Autodesk Fusion 360 part; units mm, degrees
sketch "Sketch1" plane through (0, 0, 0) normal (0, 0, 1) x (1, 0, 0)
  line L0 (-44, 15.5) -> (44, 15.5)
  line L1 (44, 15.5) -> (44, -15.5)
  line L2 (-44, -15.5) -> (-44, 15.5)
  line L3 (-44, 15.5) -> (44, -15.5) construction
  line L4 (44, 15.5) -> (-44, -15.5) construction
  circle A0 centre (-25, 0) radius 5
  circle A1 centre (25, 0) radius 5
  line L5 (-44, -15.5) -> (-44, -38.5)
  line L6 (44, -38.5) -> (44, -15.5)
  line L7 (-44, 15.5) -> (44, 15.5)
  line L8 (44, 15.5) -> (44, 28.5)
  line L9 (44, 28.5) -> (-44, 28.5)
  line L10 (-44, 28.5) -> (-44, 15.5)
  line L11 (0, -51.5) -> (-5, -51.5)
  line L12 (0, -51.5) -> (5, -51.5)
  line L13 (-5, -51.5) -> (-5, 15.5)
  line L14 (5, -51.5) -> (5, 15.5)
  line L15 (-37.3007, -49.8711) -> (-10.3733, -67.4184)
  line L16 (37.3007, -49.8711) -> (10.3733, -67.4184)
  arc A2 (-10.3733, -67.4184) -> (10.3733, -67.4184) centre (0, -51.5) ccw
  arc A3 (37.3007, -49.8711) -> (44, -38.5) centre (31, -38.5) ccw
  arc A4 (-44, -38.5) -> (-37.3007, -49.8711) centre (-31, -38.5) ccw
  dimension "d1" = 31
  dimension "d2" = 88
  dimension "d3" = 10
  dimension "d4" = 10
  dimension "d5" = 50
  dimension "d6" = 19
  dimension "d7" = 19
  dimension "d9" = 38
  dimension "d12" = 13
  dimension "d13" = 5
  dimension "d14" = 5
  dimension "d15" = 26
  dimension "d16" = 26
extrude "Extrude1" add sketch "Sketch1" along normal blind 10 contours L0 L1 L2 L5 L6 L7 L11 L12 L13 L14 L15 L16 A2 A3 A4
extrude "Extrude2" add sketch "Sketch1" along normal blind 50 contours L0 L7 L8 L9 L10
extrude "Extrude3" add sketch "Sketch1" along normal blind 50 contours L0 L7 L11 L12 L13 L14
sketch "Sketch2" plane through (0, 0, 50) normal (0, 0, 1) x (-1, 0, 0)
  line L0 (44, -28.5) -> (44, -15.5)
  line L1 (44, -15.5) -> (5, -15.5)
  line L2 (5, -15.5) -> (5, 51.5)
  line L3 (5, 51.5) -> (-5, 51.5)
  line L4 (-5, 51.5) -> (-5, -15.5)
  line L5 (-5, -15.5) -> (-44, -15.5)
  line L6 (-44, -15.5) -> (-44, -28.5)
  line L7 (-44, -28.5) -> (44, -28.5)
  circle A0 centre (19, -18.5) radius 3
  circle A1 centre (-19, -18.5) radius 3
  line L8 (19, -18.5) -> (44, -18.5)
  line L9 (-19, -18.5) -> (-44, -18.5)
  line L10 (44, -18.5) -> (44, -15.5)
  line L11 (19, -15.5) -> (19, -18.5)
  line L12 (-19, -18.5) -> (-19, -15.5)
  line L13 (-19, -18.5) -> (-19, -15.5)
  line L14 (-44, -15.5) -> (-44, -18.5)
  line L15 (44, -18.5) -> (44, -37.5)
  line L16 (44, -37.5) -> (-44, -37.5)
  line L17 (-44, -37.5) -> (-44, -18.5)
  circle A2 centre (0, -37.5) radius 9.5
  circle A3 centre (0, -37.5) radius 19
  arc A4 (24.2693, -37.5) -> (18.4447, -42.06) centre (24.2693, -43.5) ccw
  arc A5 (-18.4447, -42.06) -> (-24.2693, -37.5) centre (-24.2693, -43.5) ccw
  dimension "d23" = 6
  dimension "d24" = 6
  dimension "d25" = 38
  dimension "d26" = 25
  dimension "d31" = 19
  dimension "d32" = 19
  dimension "d33" = 38
  dimension "d35" = 12
  dimension "d36" = 12
extrude "Extrude4" cut sketch "Sketch2" against normal blind 40 contours L0 L1 A0 L8 L10
extrude "Extrude5" cut sketch "Sketch2" against normal blind 40 contours L5 L6 A1 L9 L14
sketch "Sketch3" plane through (0, 0, 50) normal (0, 0, 1) x (-1, 0, 0)
extrude "Extrude6" add sketch "Sketch2" against normal blind 50 contours L7 L15 L16 A3 | L7 L16 A2 A3 | L16 A2 A3 | L16 A3 A4 | L7 L16 L17 A3 | L7 L16 A2 A3 | L16 A3 A5
sketch "Sketch4" plane through (-5, 0, 0) normal (-1, 0, 0) x (0, -1, 0)
  line L0 (-15.5, 10) -> (51.5, 10)
  line L1 (51.5, 10) -> (51.5, 50)
  line L2 (51.5, 50) -> (-15.5, 50)
  line L3 (-15.5, 50) -> (-15.5, 10)
  line L4 (-15.5, 50) -> (51.5, 10)
extrude "Extrude7" cut sketch "Sketch4" against normal blind 85 contours L1 L2 L4
equation "d6 = ( ( 88 - 50 ) / 2 ) * 1 mm"
equation "d9 = ( 19 * 2 ) * 1 mm"
equation "d26 = ( ( 88 - 38 ) / 2 ) * 1 mm"
equation "d33 = ( 19 * 2 ) * 1 mm"
Build history of the part. All positions in model axes, mm. A direction names the side the tool comes from. Coordinates: 2 decimals unless noted, no trailing zeros. Order: outer loops, then holes, each group sorted by start corner. A loop starts at its lowest first (then second) coordinate and runs counter-clockwise, first axis right, second up. Notation, with made-up numbers: (84, 20) - (122, 20) arc R35 ccw to (122, 56) - close; hole circle Ø5 at (13, 43.25). An arc over 180 degrees is marked (long way). Put each result on its own line as item: value.
1. Saw through at C-C (z = 31.5). Write the cut outline in (x, y).
Answer sheet:
outline: (-44, 18.5) - (-22, 18.5) arc R3 ccw to (-19, 15.5) - (-5, 15.5) - (-5, -15.49) - (5, -15.49) - (5, 15.5) - (19, 15.5) arc R3 ccw to (22, 18.5) - (44, 18.5) - (44, 37.5) - (24.27, 37.5) arc R6 cw to (18.44, 42.06) arc R19 ccw to (-18.44, 42.06) arc R6 cw to (-24.27, 37.5) - (-44, 37.5) - close; hole (-3.04, 28.5) - (3.04, 28.5) arc R9.5 ccw (long way) to start
2. Pull direction Y, two halves, no side cores. Call faces 5 (the face through (20, 0, 5)), 6 (the face through (33, 18.5, 30)), 7 (the face through (-1, 27, 50)): pulls with the +Y half, pulls with the -Y half, needs draft (parallel to the pull), parting line crosses it, or undercut.
Answer sheet:
face 5: undercut
face 6: pulls with the -Y half
face 7: needs draft
3. Probe line 1 along Y through (x, z) = (38, 41); line 2 along X through (y, z) = (8.5, 19.5); line 3 along Y through (x, z) = (-25, 2.5). List the from-to ranges inside material, lowest first. Write a range as [from, to].
Answer sheet:
line 1: y = [18.5, 37.5]
line 2: x = [-5, 5]
line 3: y = [-57.89, -5], [5, 37.5]
4. Saw through at B-B (y = 0). Write the cut outline in (x, z), and give its area (3 significant figures).
Answer sheet:
outline: (-44, 0) - (-30, 0) - (-30, 10) - (-44, 10) - close; (-20, 0) - (20, 0) - (20, 10) - (5, 10) - (5, 40.75) - (-5, 40.75) - (-5, 10) - (-20, 10) - close; (30, 0) - (44, 0) - (44, 10) - (30, 10) - close
area: 987 mm^2
5. Saw through at A-A (x = 0). Write the cut outline in (y, z), and give its area (4 significant figures).
Answer sheet:
outline: (-70.5, 0) - (28.5, 0) - (28.5, 50) - (15.5, 50) - (-51.5, 10) - (-70.5, 10) - close; (47, 0) - (56.5, 0) - (56.5, 50) - (47, 50) - close
area: 3,325 mm^2
6. Saw through at D-D (y = 39). Write the cut outline in (x, z).
Answer sheet:
outline: (-20.3, 0) - (-9.38, 0) - (-9.38, 50) - (-20.3, 50) - close; (9.38, 0) - (20.3, 0) - (20.3, 50) - (9.38, 50) - close
7. Drop flat-ended pins along their axis: P1, Ø24.5, axis at x = 0, y = 37.5, coming from the +Z side; P2, Ø20, axis at y = -9, z = 33.5, coming from the -X side; P3, Ø10, axis at x = 25, y = 4.5, coming from the +Z side; P4, Ø6.5, axis at x = 0.5, z = 26, coming from the +Y side. Give the stop position or say it passes through.
Answer sheet:
P1: stops at z = 50
P2: stops at x = -5
P3: stops at z = 10
P4: stops at y = 56.5
8. Tool access for faces 1 (the face through (9, -25, 10)), 2 (the face through (21.1, 16.36, 30.28)), 3 (the face through (-21.14, 16.4, 30.28)), 4 (the face through (0, 28.5, 25)): list every direction of +Z, -Z, +X, -X, +Y, -Y with a clear straight run to the whole face (end or side of a thin tool).
Answer sheet:
face 1: +Z, -Y
face 2: +Z, +X, -Y
face 3: +Z, -X, -Y
face 4: +Z, -Z
